Drawing for the job (mm, zero at the part's lowest x, y, z). Round coordinates to 2 decimals unless told otherwise and drop trailing zeros. Loops run counter-clockwise (first coordinate to the right, second up) from the corner with the lowest first, then second, coordinate; pieces in that order, holes last. Notation, with made-up numbers: M 85.25,29.5 L 144.25,29.5 A20 cw 144.25,44.5 Z; hole C -3,72.5 d9. An arc over 180 degrees is marked long. Answer in a Markdown table with one row per item.
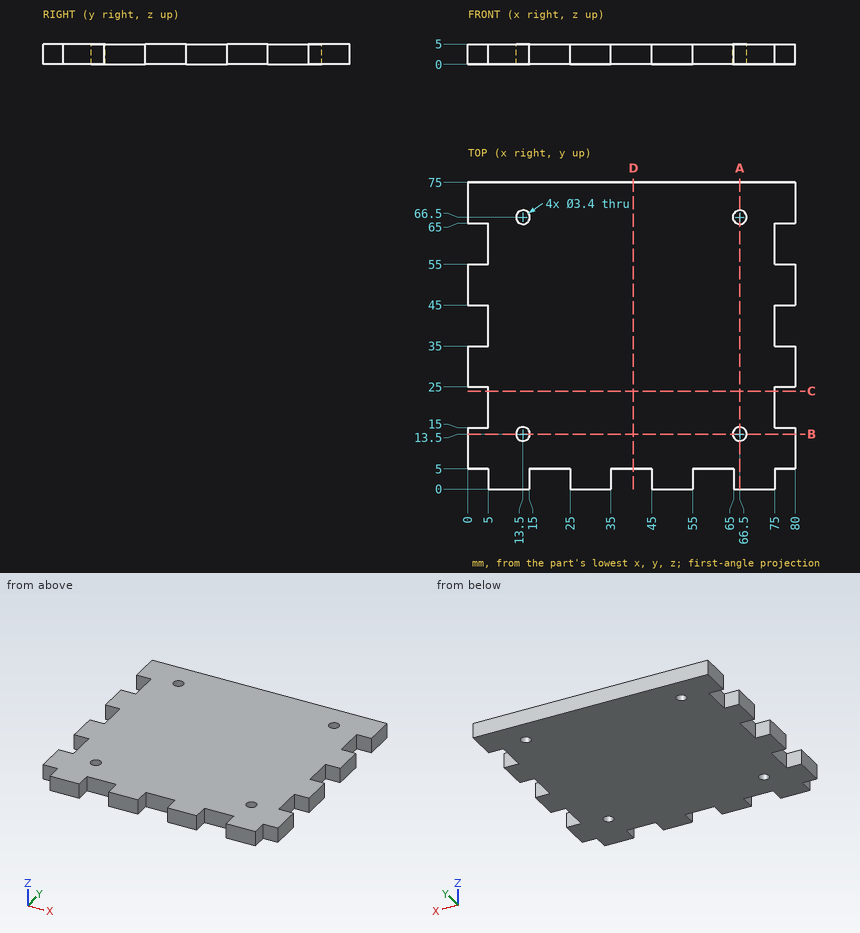
1. Pin check, flat tips, straight feed: pin 1 (2.5 mm diameter, centred on y = 3.5, z = 1.5, fed in from -X); pin 2 (2.5 mm diameter, centred on x = 41, z = 1.5, fed in from -Y); pin 3 (3 mm diameter, centred on x = 13.5, y = 66.5, fed in from +Z); pin 4 (1.5 mm diameter, centred on y = 2, z = 3.5, fed in from +X). Stop position of each tip, or through.
Verdict:
| item | result |
|---|---|
| pin 1 | stops at x = 5 |
| pin 2 | stops at y = 5 |
| pin 3 | passes through |
| pin 4 | stops at x = 75 |
2. Saw through at C-C (y = 24). Write the cut outline in (x, z), and give its area (3 significant figures).
Verdict:
| item | result |
|---|---|
| outline | M 5,0 L 75,0 L 75,5 L 5,5 Z |
| area | 350 mm² |
3. Wall check: probe 1 along Y at (x, z) = (13.5, 1.75); probe 2 along X at (y, z) = (66.5, 1); probe 3 along X at (y, z) = (41, 0.45). Give the ranges that are in metal, low to high.
Verdict:
| item | result |
|---|---|
| probe 1 | y = 0 to 11.8, 15.2 to 64.8, 68.2 to 75 |
| probe 2 | x = 0 to 11.8, 15.2 to 64.8, 68.2 to 80 |
| probe 3 | x = 5 to 75 |
4. Saw through at A-A (x = 66.5). Write the cut outline in (y, z).
Verdict:
| item | result |
|---|---|
| outline | M 0,0 L 11.8,0 L 11.8,5 L 0,5 Z; M 15.2,0 L 64.8,0 L 64.8,5 L 15.2,5 Z; M 68.2,0 L 75,0 L 75,5 L 68.2,5 Z |
5. Saw through at B-B (y = 13.5). Write the cut outline in (x, z), and give its area (3 significant figures).
Verdict:
| item | result |
|---|---|
| outline | M 0,0 L 11.8,0 L 11.8,5 L 0,5 Z; M 15.2,0 L 64.8,0 L 64.8,5 L 15.2,5 Z; M 68.2,0 L 80,0 L 80,5 L 68.2,5 Z |
| area | 366 mm² |
